```python
from build123d import *

# Parameters (mm, degrees)
SKETCH1_R             = 2.1
BOSS_EXTRUDE1_DEPTH   = 3
BOSS_EXTRUDE1_2_DEPTH = 3
BOSS_EXTRUDE1_3_DEPTH = 3
SKETCH1_W             = 100
SKETCH1_H             = 120
BOSS_EXTRUDE1_4_DEPTH = 3
SKETCH2_R             = 2.1
CUT_EXTRUDE1_DEPTH    = 10
SKETCH3_W             = 100
SKETCH3_H             = 3
BOSS_EXTRUDE2_DEPTH   = 160
SKETCH4_R             = 3
SKETCH4_R_2           = 2.1
CUT_EXTRUDE2_DEPTH    = 160
SKETCH5_R             = 2.1
CUT_EXTRUDE3_DEPTH    = 10


with BuildPart() as part:
    # Sketch1 → Boss-Extrude1 (new body)
    with BuildSketch(Plane(origin=(0, 0, 0), x_dir=(1, 0, 0), z_dir=(0, 1, 0))):
        with Locations(Location((-42, 70, 0), (0, 0, 270))):
            Circle(SKETCH1_R)
    extrude(amount=BOSS_EXTRUDE1_DEPTH)


with BuildPart() as body_2:
    # Sketch1 → Boss-Extrude1 2 (new body)
    with BuildSketch(Plane(origin=(0, 0, 0), x_dir=(1, 0, 0), z_dir=(0, 1, 0))):
        with Locations(Location((0, 70, 0), (0, 0, 270))):
            Circle(SKETCH1_R)
    extrude(amount=BOSS_EXTRUDE1_2_DEPTH)


with BuildPart() as body_3:
    # Sketch1 → Boss-Extrude1 3 (new body)
    with BuildSketch(Plane(origin=(0, 0, 0), x_dir=(1, 0, 0), z_dir=(0, 1, 0))):
        with Locations(Location((42, 70, 0), (0, 0, 270))):
            Circle(SKETCH1_R)
    extrude(amount=BOSS_EXTRUDE1_3_DEPTH)


with BuildPart() as body_4:
    # Sketch1 → Boss-Extrude1 4 (new body)
    with BuildSketch(Plane(origin=(0, 0, 0), x_dir=(1, 0, 0), z_dir=(0, 1, 0))):
        Rectangle(SKETCH1_W, SKETCH1_H)
        with Locations(Location((41.5, -50, 0), (0, 0, 90))):
            Circle(SKETCH1_R, mode=Mode.SUBTRACT)
        with Locations(Location((-41.5, -50, 0), (0, 0, 270))):
            Circle(SKETCH1_R, mode=Mode.SUBTRACT)
    extrude(amount=BOSS_EXTRUDE1_4_DEPTH)

    # Sketch2 → Cut-Extrude1 (cut)
    with BuildSketch(Plane.XZ):
        with Locations(Location((24.5, 50, 0), (0, 0, 270))):
            Circle(SKETCH2_R)
        with Locations(Location((-24.5, 50, 0), (0, 0, 270))):
            Circle(SKETCH2_R)
    extrude(amount=-CUT_EXTRUDE1_DEPTH, mode=Mode.SUBTRACT)

    # Sketch3 → Boss-Extrude2 (add)
    with BuildSketch(Plane(origin=(0, 0, -60), x_dir=(-1, 0, 0), z_dir=(0, 0, -1))):
        with Locations((0, 1.5)):
            Rectangle(SKETCH3_W, SKETCH3_H)
    extrude(amount=BOSS_EXTRUDE2_DEPTH)

    # Sketch4 → Cut-Extrude2 (cut)
    with BuildSketch(Plane.XZ):
        with Locations(Location((17.5, -206.7, 0), (0, 0, 270))):
            Circle(SKETCH4_R)
        with Locations(Location((-17.5, -206.7, 0), (0, 0, 270))):
            Circle(SKETCH4_R)
        with Locations(Location((-41.5, -170, 0), (0, 0, 270))):
            Circle(SKETCH4_R_2)
        with Locations(Location((41.5, -170, 0), (0, 0, 270))):
            Circle(SKETCH4_R_2)
    extrude(amount=-CUT_EXTRUDE2_DEPTH, mode=Mode.SUBTRACT)


with BuildPart() as cut_extrude3_tool:
    # Sketch5 → Cut-Extrude3 (new body)
    with BuildSketch(Plane.XZ):
        with Locations(Location((-42, -70, 0), (0, 0, 270))):
            Circle(SKETCH5_R)
        with Locations(Location((0, -70, 0), (0, 0, 270))):
            Circle(SKETCH5_R)
        with Locations(Location((42, -70, 0), (0, 0, 270))):
            Circle(SKETCH5_R)
    extrude(amount=-CUT_EXTRUDE3_DEPTH)


with BuildPart() as part_1:
    add(part.part)

    # Cut-Extrude3: cut by cut_extrude3_tool
    add(cut_extrude3_tool.part, mode=Mode.SUBTRACT)


with BuildPart() as body_2_1:
    add(body_2.part)

    # Cut-Extrude3: cut by cut_extrude3_tool
    add(cut_extrude3_tool.part, mode=Mode.SUBTRACT)


with BuildPart() as body_3_1:
    add(body_3.part)

    # Cut-Extrude3: cut by cut_extrude3_tool
    add(cut_extrude3_tool.part, mode=Mode.SUBTRACT)


with BuildPart() as body_4_1:
    add(body_4.part)

    # Cut-Extrude3: cut by cut_extrude3_tool
    add(cut_extrude3_tool.part, mode=Mode.SUBTRACT)


solid = body_4_1.part
```
The model under review builds one solid part; all positions refer to its coordinate system, in mm. Round coordinates to 2 decimals unless told otherwise and drop trailing zeros. Order: outer loops, then holes, each group sorted by start corner. A loop starts at its lowest first (then second) coordinate and runs counter-clockwise, first axis right, second up. Notation, with made-up numbers: (-39.75, 0) -> (4.25, 0) arc R35 cw to (4.25, 32) -> close; hole circle Ø10 at (-4.5, -18). An arc over 180 degrees is marked (long way). One line per item, written item: value. Start each with the question number.
Q1. Take a section at A-A (x = -17.5). Write out the cut boundary in (y, z).
Q2. Wall thickness on line 1 (X direction, y = 2.05, z = 50); line 2 (X direction, y = 1, z = -70); line 3 (Z direction, x = 19, y = 0.85): over which ranges is each line inside the solid? List them lowest first.
Q3. Clearance check with a flat-ended pin moving along its axis: pin 1 Ø5 at (x, z) = (17.5, -206.7) entering from +Y. State where the tip first meets the part, or that it passes through.
Q4. Mouldability with a two-part tool opening along Z and no side actions: class faces 1 (the face through (1, 0, -78)), 2 (the face through (-16.6, 1.48, -209.56)) as released by +Z, released by -Z, zero draft, split by the parting line, or undercut.
Reported:
1. outline: (0, -220) -> (3, -220) -> (3, -209.7) -> (0, -209.7) -> close; (0, -203.7) -> (3, -203.7) -> (3, 60) -> (0, 60) -> close
2. line 1: x = -50 to -43.6, -39.4 to -26.6, -22.4 to 22.4, 26.6 to 39.4, 43.6 to 50
2. line 2: x = -50 to -44.1, -39.9 to -2.1, 2.1 to 39.9, 44.1 to 50
2. line 3: z = -220 to -209.3, -204.1 to 60
3. pin 1: passes through
4. face 1: zero draft
4. face 2: undercut
